```python
from build123d import *

# Parameters (mm, degrees)
F2_R     = 2.6
F3_DEPTH = 6
F4_R     = 4
F5_DEPTH = 28.401


with BuildPart() as f1:
    # F0 (on Front) → F1 (revolve)
    with BuildSketch(Plane.XZ):
        Polygon((0, 28.4), (0, 8), (26.4, 8), (26.4, 18.5), (6, 18.5), (6, 28.4), align=None)
    revolve(axis=Axis((58.458176, 0, 0), (1, 0, 0)))

    # F2 (on Right) → F3 (cut, through all)
    with BuildSketch(Plane.YZ):
        with Locations((11.875, 20.568103)):
            Circle(F2_R)
        with Locations((23.75, 0)):
            Circle(F2_R)
        with Locations((11.875, -20.568103)):
            Circle(F2_R)
        with Locations((-11.875, -20.568103)):
            Circle(F2_R)
        with Locations((-23.75, 0)):
            Circle(F2_R)
        with Locations((-11.875, 20.568103)):
            Circle(F2_R)
    extrude(amount=F3_DEPTH, mode=Mode.SUBTRACT)

    # F4 (on Top) → F5 (cut, through all)
    with BuildSketch(Plane.XY):
        with Locations((16.2, 0)):
            Circle(F4_R)
    extrude(amount=-F5_DEPTH, mode=Mode.SUBTRACT)


solid = f1.part
```
The model under review builds one solid part; all positions refer to its coordinate system, in mm. A direction names the side the tool comes from. Coordinates: 2 decimals unless noted, no trailing zeros. Write each loop counter-clockwise with the first axis right and the second up, starting at its lowest first coordinate (ties: lowest second). Pieces come first, ordered by that corner, then holes. Notation, with made-up numbers: (-2, 23.5) - (47, 23.5) arc R20 cw to (47, 58.5) - close; hole circle Ø7 at (69, -7). An arc over 180 degrees is marked (long way). Answer in a Markdown table with one row per item. Add a question column.
Q1. For faces 1 (the face through (19.895, -1.532, -12.633)), 2 (the face through (2.958, 14.355, -19.787)), 3 (the face through (6, 19, 0)), list the 3-axis set-ups (+Z, -Z, +X, -X, +Y, -Y) from which the entire face can be reached by the end or side of a thin tool; tool diameter is ignored.
Q2. Consider section D-D on x = 21.25. Give the boundary of the cut face in (y, z).
Q3. Draft analysis for pull direction Z (two halves, no side actions). For faces 4 (the face through (2.96, -21.27, 0.78)), 5 (the face through (0, 6, 6)), 6 (the face through (2.958, -28.158, -3.697)), state which applies: +Z half, -Z half, draft (parallel to the pull), parting line (faces both ways), or undercut.
Q4. To check wall thickness, follow line 1 along Y through (x, z) = (15, 0); line 2 along X through (y, z) = (0, -13). State the ranges of each line that lie inside material, in increasing order. Write a range as from..to.
Q5. Clearance check with flat-ended pins moving along their axes: pin 1 (10 mm diameter, centred on x = 10.5, z = 12.5, fed in from +Y); pin 2 (6 mm diameter, centred on y = 23.75, z = 0, fed in from +X); pin 3 (4.5 mm diameter, centred on y = -23.75, z = 0, fed in from -X); pin 4 (1.5 mm diameter, centred on x = 5.5, z = -22.5, fed in from +Y). State where each tip first meets the part, or that it passes through.
Q6. Consider section A-A on y = 0. Give the boundary of the cut face in (x, z).
Q7. Consider section B-B on z = 0. Give the boundary of the cut face in (x, y).
Q8. Consider section C-C on y = -23.75. Give the boundary of the cut face in (x, z), then the cut area to 3 significant figures.
Answers below:
| question | item | result |
|---|---|---|
| 1 | face 1 | -Z |
| 1 | face 2 | +X, -X |
| 1 | face 3 | +X |
| 2 | outline | circle Ø37 at (0, 0); hole circle Ø16 at (0, 0) |
| 3 | face 4 | undercut |
| 3 | face 5 | draft |
| 3 | face 6 | parting line |
| 4 | line 1 | -18.5..-8, 8..18.5 |
| 4 | line 2 | 0..12.2, 20.2..26.4 |
| 5 | pin 1 | y = 26.46 |
| 5 | pin 2 | x = 6 |
| 5 | pin 3 | through |
| 5 | pin 4 | y = 18.26 |
| 6 | outline | (0, -28.4) - (6, -28.4) - (6, -18.5) - (12.2, -18.5) - (12.2, -8) - (0, -8) - close; (0, 8) - (26.4, 8) - (26.4, 18.5) - (6, 18.5) - (6, 28.4) - (0, 28.4) - close; (20.2, -18.5) - (26.4, -18.5) - (26.4, -8) - (20.2, -8) - close |
| 7 | outline | (0, -28.4) - (6, -28.4) - (6, -26.35) - (0, -26.35) - close; (0, -21.15) - (6, -21.15) - (6, -18.5) - (26.4, -18.5) - (26.4, -8) - (0, -8) - close; (0, 8) - (26.4, 8) - (26.4, 18.5) - (6, 18.5) - (6, 21.15) - (0, 21.15) - close; (0, 26.35) - (6, 26.35) - (6, 28.4) - (0, 28.4) - close |
| 8 | outline | (0, -15.57) - (6, -15.57) - (6, -2.6) - (0, -2.6) - close; (0, 2.6) - (6, 2.6) - (6, 15.57) - (0, 15.57) - close |
| 8 | area | 156 mm² |
